Verification items for the finished model (mm, model axes). Coordinates: 2 decimals unless noted, no trailing zeros. Write each loop counter-clockwise with the first axis right and the second up, starting at its lowest first coordinate (ties: lowest second). Pieces come first, ordered by that corner, then holes. Notation, with made-up numbers: (-16, -21.5) -> (36, -21.5) arc R24 cw to (36, -11.5) -> close; hole circle Ø5 at (82, 86.25). An arc over 180 degrees is marked (long way). Use CSV: the item, a comma, the result in double quotes.
```python
from build123d import *

# Parameters (mm, degrees)
SKETCH_1_W          = 84
SKETCH_1_H          = 100
EXTRUDE_1_DEPTH     = 3
SKETCH_3_R          = 3
CUT_EXTRUDE_1_DEPTH = 3
SKETCH_4_W          = 3
SKETCH_4_H          = 100
EXTRUDE_2_DEPTH     = 2
SKETCH_5_R          = 1.6
CUT_EXTRUDE_2_DEPTH = 4


with BuildPart() as part:
    # 草图1 → 凸台-拉伸1 (new body)
    with BuildSketch(Plane.XY):
        with Locations((42, 50)):
            Rectangle(SKETCH_1_W, SKETCH_1_H)
    extrude(amount=EXTRUDE_1_DEPTH)

    # 草图3 → 切除-拉伸1 (cut)
    with BuildSketch(Plane.XY.offset(3)):
        with Locations((42, 31.24)):
            Circle(SKETCH_3_R)
        with Locations((42, 56.24)):
            Circle(SKETCH_3_R)
    extrude(amount=-CUT_EXTRUDE_1_DEPTH, mode=Mode.SUBTRACT)

    # 草图4 → 凸台-拉伸2 (add)
    with BuildSketch(Plane.ZY):
        with Locations((1.5, 50)):
            Rectangle(SKETCH_4_W, SKETCH_4_H)
    extrude(amount=EXTRUDE_2_DEPTH)

    # 草图5 → 切除-拉伸2 (cut, through all)
    with BuildSketch(Plane.XY.offset(3)):
        with Locations((82, 10)):
            Circle(SKETCH_5_R)
        with Locations((82, 90)):
            Circle(SKETCH_5_R)
        with Locations((0, 90)):
            Circle(SKETCH_5_R)
        with Locations((0, 10)):
            Circle(SKETCH_5_R)
    extrude(amount=-CUT_EXTRUDE_2_DEPTH, mode=Mode.SUBTRACT)


solid = part.part
```
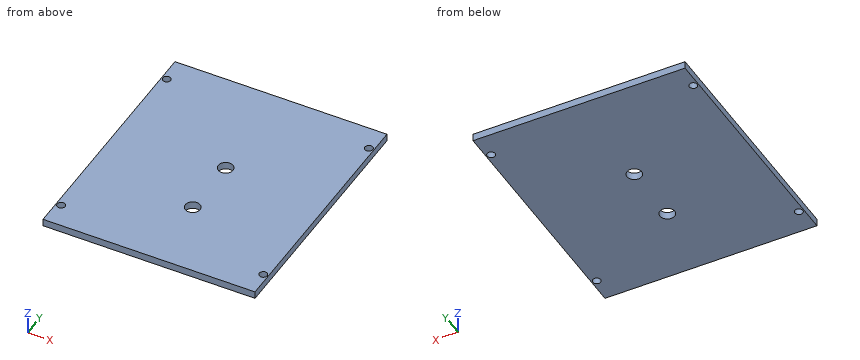
1) Gauge pin test, flat end, axial feed: pin 1 (2.5 mm diameter, centred on x = 82, y = 90, fed in from -Z). Record the tip position at first contact, or that the pin passes through.
Return value:
pin 1,"through"
2) Cross-section at C-C (x = 42). Record the boundary of the cut face in (y, z), plus the area to 3 significant figures.
Return value:
outline,"(0, 0) -> (28.24, 0) -> (28.24, 3) -> (0, 3) -> close; (34.24, 0) -> (53.24, 0) -> (53.24, 3) -> (34.24, 3) -> close; (59.24, 0) -> (100, 0) -> (100, 3) -> (59.24, 3) -> close"
area,"264 mm2"
3) Scan lines: L1, parallel to Y at x = 82, z = 0.6; L2, parallel to X at y = 90, z = 1.1; L3, parallel to X at y = 34, z = 0.65. Record each from-to range of solid material in increasing order.
Return value:
L1,"0 to 8.4, 11.6 to 88.4, 91.6 to 100"
L2,"-2 to -1.6, 1.6 to 80.4, 83.6 to 84"
L3,"-2 to 40.82, 43.18 to 84"
4) Cross-section at A-A (y = 56.24). Record the boundary of the cut face in (x, z).
Return value:
outline,"(-2, 0) -> (39, 0) -> (39, 3) -> (-2, 3) -> close; (45, 0) -> (84, 0) -> (84, 3) -> (45, 3) -> close"
5) Cross-section at B-B (x = 0). Record the boundary of the cut face in (y, z).
Return value:
outline,"(0, 0) -> (8.4, 0) -> (8.4, 3) -> (0, 3) -> close; (11.6, 0) -> (88.4, 0) -> (88.4, 3) -> (11.6, 3) -> close; (91.6, 0) -> (100, 0) -> (100, 3) -> (91.6, 3) -> close"
